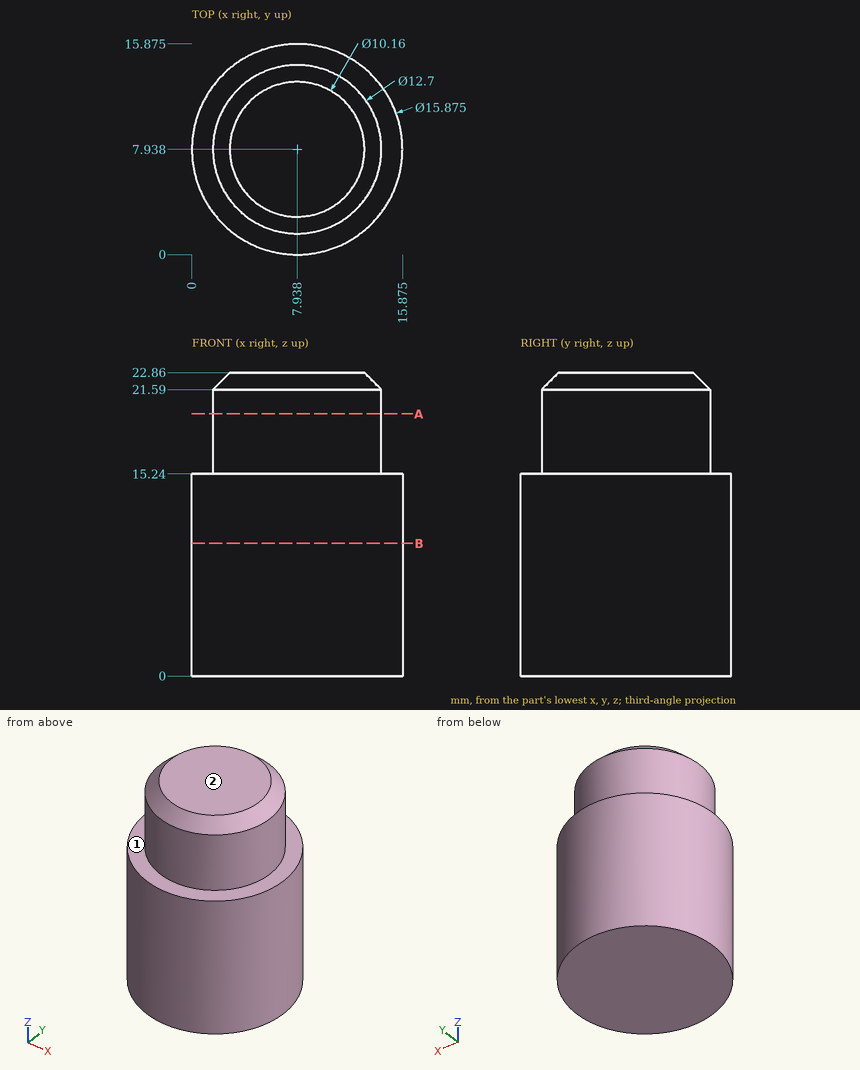
Input: dimensioned drawing with shaded views. Units: mm. Origin: part minimum x, y, z. A direction names the side the tool comes from. Coordinates: 2 decimals unless noted, no trailing zeros. Order: outer loops, then holes, each group sorted by start corner. A loop starts at its lowest first (then second) coordinate and runs counter-clockwise, first axis right, second up.
(1) Access query for the marked faces 1 and 2. Directions: +Z, -Z, +X, -X, +Y, -Y. A direction counts if a zero-diameter tool reaches every point of the face in a straight line with its end or side. Return the directions, or none.
(2) Section query B-B (z = 10). Return the cut outline in (x, y) (1 decimal), plus the area to 3 significant figures.
(3) Material intervals for probe 1 along Z at (x, y) = (1.5, 9.25); probe 2 along Y at (x, z) = (7.75, 19) (1 decimal); probe 3 along X at (y, z) = (7.75, 10), sorted ascending.
(4) Section query A-A (z = 19.75). Return the cut outline in (x, y).
(5) First-contact query: pin 1 (2 mm diameter, centred on y = 11.5, z = 5, fed in from -X) (1 decimal); pin 2 (1.5 mm diameter, centred on y = 9.5, z = 7.5, fed in from +X); pin 3 (1.5 mm diameter, centred on x = 11.5, z = 4, fed in from +Y); pin 4 (6 mm diameter, centred on x = 1.5, y = 10, fed in from +Z). Flat tips, straight axial feed; report the tip coordinate or a pass-through.
Solution:
1. face 1: +Z
1. face 2: +Z, +X, -X, +Y, -Y
2. outline: circle Ø15.9 at (7.9, 7.9)
2. area: 198 mm2
3. probe 1: z = 0 to 15.24
3. probe 2: y = 1.6 to 14.3
3. probe 3: x = 0 to 15.87
4. outline: circle Ø12.7 at (7.94, 7.94)
5. pin 1: stops at x = 0.4
5. pin 2: stops at x = 15.83
5. pin 3: stops at y = 15.36
5. pin 4: stops at z = 22.86
